Design review of the part built by this model. Coordinates are the model's own, in mm. A direction names the side the tool comes from. Give positions to 0.01 mm unless a question says otherwise; leave off trailing zeros. Order: outer loops, then holes, each group sorted by start corner. A loop starts at its lowest first (then second) coordinate and runs counter-clockwise, first axis right, second up.
```python
from build123d import *

# Parameters (mm, degrees)
CROQUIS1_R                 = 13
CROQUIS1_R_2               = 11.05
SALIENTE_EXTRUIR1_DEPTH    = 1
BARRER_L_MINA1_PROFILE_R   = 13.05
BARRER_L_MINA1_PROFILE_R_2 = 11.05


with BuildPart() as part:
    # Croquis1 → Saliente-Extruir1 (new body)
    with BuildSketch(Plane(origin=(0, 0, 0), x_dir=(1, 0, 0), z_dir=(0, 1, 0))):
        with Locations(Location((0, 0, 0), (0, 0, 270))):
            Circle(CROQUIS1_R)
        with Locations(Location((0, 0, 0), (0, 0, 270))):
            Circle(CROQUIS1_R_2, mode=Mode.SUBTRACT)
    extrude(amount=SALIENTE_EXTRUIR1_DEPTH)

    # Barrer-L_mina1: sweep along a path in Croquis2
    with BuildLine(Plane.XY) as barrer_l_mina1_path:
        Line((0, 1), (0, 21))
        ThreePointArc((0, 21), (-7.11124406, 33.758037847), (-21.702337296, 34.41933958))
        Line((-21.702337296, 34.41933958), (-40.489412708, 25.036067367))
    # Barrer-L_mina1 profile (on start of the path) → Barrer-L_mina1 (sweep)
    with BuildSketch(Plane.ZX.offset(1)):
        Circle(BARRER_L_MINA1_PROFILE_R)
        Circle(BARRER_L_MINA1_PROFILE_R_2, mode=Mode.SUBTRACT)
    sweep(path=barrer_l_mina1_path.line)


solid = part.part
```
1. Take a section at C-C (y = 16). State how many separate pieces and enclosed holes the cut face has, then the cut area to 3 significant figures.
Recorded:
separate pieces: 2
enclosed holes: 1
area: 213 mm2
2. Take a section at A-A (z = 0). State the section outline as (x, y) points, then the cut area to 3 significant figures.
Recorded:
outline: (-46.32, 36.71) - (-45.43, 34.92) - (-26.64, 44.3) arc R26.05 cw to (11.05, 21) - (11.05, 0) - (13, 0) - (13, 1) - (13.05, 1) - (13.05, 21) arc R28.05 ccw to (-27.53, 46.09) - close; (-35.55, 15.15) - (-34.66, 13.36) - (-15.87, 22.74) arc R1.95 cw to (-13.05, 21) - (-13.05, 1) - (-13, 1) - (-13, 0) - (-11.05, 0) - (-11.05, 21) arc R3.95 ccw to (-16.76, 24.53) - close
area: 290 mm2
3. Take a section at B-B (z = 10.25). State the section outline as (x, y) points, then the cut area to 3 significant figures.
Recorded:
outline: (-44.1, 32.26) - (-42.33, 28.73) - (-23.55, 38.11) arc R19.13 cw to (4.13, 21) - (4.13, 0) - (8, 0) - (8, 1) - (8.08, 1) - (8.08, 21) arc R23.08 ccw to (-25.31, 41.65) - close; (-38.64, 21.34) - (-36.88, 17.81) - (-18.09, 27.19) arc R6.92 cw to (-8.08, 21) - (-8.08, 1) - (-8, 1) - (-8, 0) - (-4.13, 0) - (-4.13, 21) arc R10.87 ccw to (-19.86, 30.73) - close
area: 573 mm2
4. Draft analysis for pull direction Y (two halves, no side actions). For faces 1 (the face through (-10.787, 10.353, -2.395)), 2 (the face through (-10, 0, -6)), 3 (the face through (-34.564, 36.343, -8.144)), state which applies: pulls with the +Y half, pulls with the -Y half, needs draft (parallel to the pull), parting line crosses it, or undercut.
Recorded:
face 1: needs draft
face 2: pulls with the -Y half
face 3: undercut
5. For line 1 along X through (y, z) = (5.5, 0); line 2 along Y through (x, z) = (-23.5, -7.75); line 3 along Z through (x, y) = (-27, 23), list the stretches that pass through material, from the lowest coordinate up.
Recorded:
line 1: x = -13.05 to -11.05, 11.05 to 13.05
line 2: y = 21.79 to 24.72, 42.24 to 45.04
line 3: z = -10.43 to -7.78, 7.78 to 10.43
6. Machinability: for faces 4 (the face through (-44.836, 33.739, 5.861)), 5 (the face through (8.82, 11.14, -9.62)), which of the approach directions +Z, -Z, +X, -X, +Y, -Y give a long, thin tool a straight path to every point of the face, cutting with its end or side? Answer none if there is none.
Recorded:
face 4: +Z, -Z, -X, -Y
face 5: -Y
7. For pin 1 (4 mm diameter, centred on x = -7.5, y = 14.5, fed in from +Z); pin 2 (1.5 mm diameter, centred on x = 0.5, z = 0, fed in from +Y); pin 3 (1.5 mm diameter, centred on y = 41.5, z = -0.5, fed in from +X), all flat-tipped, find the tip position at first contact; note any pin that passes through.
Recorded:
pin 1: stops at z = 11.83
pin 2: stops at y = 44.86
pin 3: stops at x = 4.91
